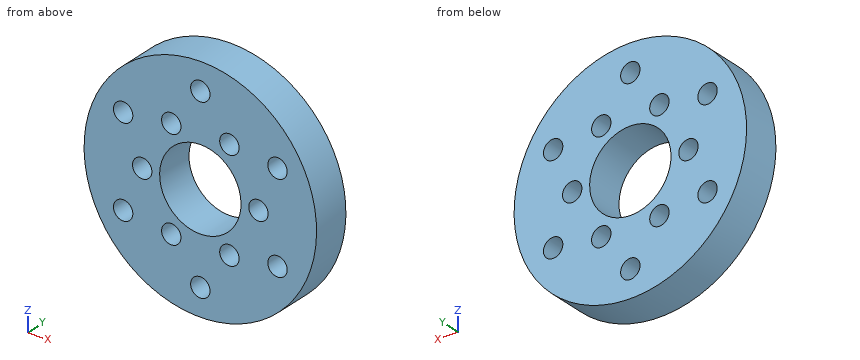
```python
from build123d import *

# Parameters (mm, degrees)
SKETCH1_R           = 30
SKETCH1_R_2         = 2.5
SKETCH1_R_3         = 10.5
BOSS_EXTRUDE1_DEPTH = 10
SKETCH2_R           = 2.5
CUT_EXTRUDE1_DEPTH  = 10


with BuildPart() as part:
    # Sketch1 → Boss-Extrude1 (new body)
    with BuildSketch(Plane(origin=(0, 0, 0), x_dir=(1, 0, 0), z_dir=(0, 1, 0))):
        with Locations(Location((0, 0, 0), (0, 0, 270))):
            Circle(SKETCH1_R)
        with Locations(Location((0, 23, 0), (0, 0, 270))):
            Circle(SKETCH1_R_2, mode=Mode.SUBTRACT)
        with Locations(Location((19.918584287, 11.5, 0), (0, 0, 270))):
            Circle(SKETCH1_R_2, mode=Mode.SUBTRACT)
        with Locations(Location((19.918584287, -11.5, 0), (0, 0, 270))):
            Circle(SKETCH1_R_2, mode=Mode.SUBTRACT)
        with Locations(Location((0, -23, 0), (0, 0, 270))):
            Circle(SKETCH1_R_2, mode=Mode.SUBTRACT)
        with Locations(Location((-19.918584287, -11.5, 0), (0, 0, 270))):
            Circle(SKETCH1_R_2, mode=Mode.SUBTRACT)
        with Locations(Location((-19.918584287, 11.5, 0), (0, 0, 270))):
            Circle(SKETCH1_R_2, mode=Mode.SUBTRACT)
        with Locations(Location((0, 0, 0), (0, 0, 270))):
            Circle(SKETCH1_R_3, mode=Mode.SUBTRACT)
    extrude(amount=BOSS_EXTRUDE1_DEPTH)

    # Sketch2 → Cut-Extrude1 (cut)
    with BuildSketch(Plane(origin=(0, 10, 0), x_dir=(1, 0, 0), z_dir=(0, 1, 0))):
        with Locations(Location((-7.5, 12.990381057, 0), (0, 0, 270))):
            Circle(SKETCH2_R)
        with Locations(Location((7.5, 12.990381057, 0), (0, 0, 270))):
            Circle(SKETCH2_R)
        with Locations(Location((15, 0, 0), (0, 0, 270))):
            Circle(SKETCH2_R)
        with Locations(Location((7.5, -12.990381057, 0), (0, 0, 270))):
            Circle(SKETCH2_R)
        with Locations(Location((-7.5, -12.990381057, 0), (0, 0, 270))):
            Circle(SKETCH2_R)
        with Locations(Location((-15, 0, 0), (0, 0, 270))):
            Circle(SKETCH2_R)
    extrude(amount=-CUT_EXTRUDE1_DEPTH, mode=Mode.SUBTRACT)


solid = part.part
```
Build history of the part. All positions in model axes, mm. Round coordinates to 2 decimals unless told otherwise and drop trailing zeros. Write each loop counter-clockwise with the first axis right and the second up, starting at its lowest first coordinate (ties: lowest second). Pieces come first, ordered by that corner, then holes. Notation, with made-up numbers: (0, 39.5) -> (43, 39.5) arc R10 ccw to (43, 47.5) -> close; hole circle Ø10 at (47.25, 38). An arc over 180 degrees is marked (long way). Put each result on its own line as item: value.
Item 1: Flat gauge pins, fed straight in: P1, Ø6, axis at x = 0, z = -23, coming from the -Y side; P2, Ø2, axis at y = 1, z = 7, coming from the -X side; P3, Ø3, axis at y = 6, z = -14, coming from the +X side; P4, Ø4.5, axis at x = 0, z = 23, coming from the +Y side. Where does each tip first touch, or does it go through?
Here are the results:
P1: stops at y = 0
P2: stops at x = -29.39
P3: stops at x = 27.27
P4: passes through
Item 2: Slice it at C-C, the plane z = 23. Give the cut face in (x, y).
Here are the results:
outline: (-19.26, 0) -> (-2.5, 0) -> (-2.5, 10) -> (-19.26, 10) -> close; (2.5, 0) -> (19.26, 0) -> (19.26, 10) -> (2.5, 10) -> close
Item 3: Slice it at B-B, the plane x = -9. Give the cut face in (y, z).
Here are the results:
outline: (0, -28.62) -> (10, -28.62) -> (10, -14.99) -> (0, -14.99) -> close; (0, -10.99) -> (10, -10.99) -> (10, -5.41) -> (0, -5.41) -> close; (0, 5.41) -> (10, 5.41) -> (10, 10.99) -> (0, 10.99) -> close; (0, 14.99) -> (10, 14.99) -> (10, 28.62) -> (0, 28.62) -> close
Item 4: Slice it at A-A, the plane z = 0.5. Give the cut face in (x, y).
Here are the results:
outline: (-30, 0) -> (-17.45, 0) -> (-17.45, 10) -> (-30, 10) -> close; (-12.55, 0) -> (-10.49, 0) -> (-10.49, 10) -> (-12.55, 10) -> close; (10.49, 0) -> (12.55, 0) -> (12.55, 10) -> (10.49, 10) -> close; (17.45, 0) -> (30, 0) -> (30, 10) -> (17.45, 10) -> close
Item 5: Slice it at D-D, the plane x = -15. Give the cut face in (y, z).
Here are the results:
outline: (0, -25.98) -> (10, -25.98) -> (10, -2.5) -> (0, -2.5) -> close; (0, 2.5) -> (10, 2.5) -> (10, 25.98) -> (0, 25.98) -> close
Item 6: Wall check: probe 1 along X at (y, z) = (3.5, 0); probe 2 along Z at (x, y) = (-6, 9.5); probe 3 along X at (y, z) = (6, 11.5). Give the ranges that are in metal, low to high. Write a range as from..to.
Here are the results:
probe 1: x = -30..-17.5, -12.5..-10.5, 10.5..12.5, 17.5..30
probe 2: z = -29.39..-14.99, -10.99..-8.62, 8.62..10.99, 14.99..29.39
probe 3: x = -27.71..-22.42, -17.42..-9.51, -5.49..5.49, 9.51..17.42, 22.42..27.71
